Input: dimensioned drawing with shaded views. Units: mm. Origin: part minimum x, y, z. Coordinates: 2 decimals unless noted, no trailing zeros. Write each loop counter-clockwise with the first axis right and the second up, starting at its lowest first coordinate (ties: lowest second). Pieces come first, ordered by that corner, then holes. Notation, with made-up numbers: M -3.5,26.25 L 0.5,26.25 A7 ccw 0.5,34.25 Z; hole C 1.25,-12.75 d3. An arc over 180 degrees is marked long. Write each question's results on one line, items separated by ' | '. Start each with the question number.
1. Section query B-B, the plane z = 200. Output: boundary loops of the cut face in (x, y).
2. Section query C-C, the plane y = 40. Output: boundary loops of the cut face in (x, z), and give its area (3 significant figures).
3. Section query D-D, the plane x = 311. Output: boundary loops of the cut face in (y, z).
4. First-contact query: pin 1 (20 mm diameter, centred on y = 31, z = 304.5, fed in from +X); pin 2 (20 mm diameter, centred on x = 307.5, y = 40, fed in from -Z); pin 3 (6 mm diameter, centred on x = 199, z = 53.5, fed in from +Y). Flat tips, straight axial feed; report the tip coordinate or a pass-through.
5. Section query A-A, the plane x = 200. Output: boundary loops of the cut face in (y, z), and give its area (3 significant figures).
6. Ray query, probe 1 along Y at (x, z) = (451.75, 200); probe 2 along Y at (x, z) = (99, 50). Return the intervals inside material, ascending.
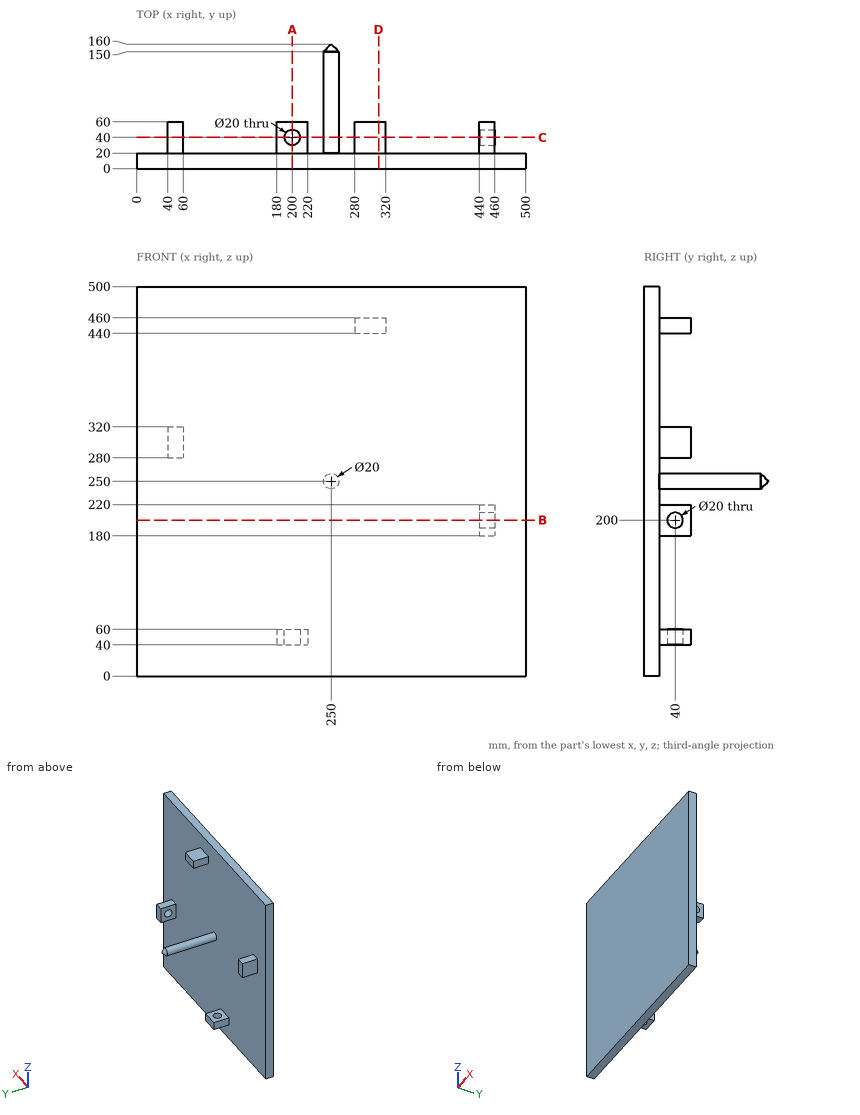
Answer:
1) outline: M 0,0 L 500,0 L 500,20 L 460,20 L 460,30 L 440,30 L 440,20 L 0,20 Z; M 440,50 L 460,50 L 460,60 L 440,60 Z
2) outline: M 40,280 L 60,280 L 60,320 L 40,320 Z; M 180,40 L 190,40 L 190,60 L 180,60 Z; M 210,40 L 220,40 L 220,60 L 210,60 Z; C 250,250 d20; M 280,440 L 320,440 L 320,460 L 280,460 Z; M 440,180 L 460,180 L 460,190 L 440,190 Z; M 440,210 L 460,210 L 460,220 L 440,220 Z | area: 2,710 mm^2
3) outline: M 0,0 L 20,0 L 20,440 L 60,440 L 60,460 L 20,460 L 20,500 L 0,500 Z
4) pin 1: x = 60 | pin 2: z = 440 | pin 3: y = 60
5) outline: M 0,0 L 20,0 L 20,40 L 30,40 L 30,60 L 20,60 L 20,500 L 0,500 Z; M 50,40 L 60,40 L 60,60 L 50,60 Z | area: 10,400 mm^2
6) probe 1: 0 to 30, 50 to 60 | probe 2: 0 to 20
